Autodesk Inventor part; units mm, degrees
ref_plane "YZ Plane" through (0, 0, 0) normal (1, 0, 0) x (0, 1, 0)
ref_plane "XZ Plane" through (0, 0, 0) normal (0, 1, 0) x (-1, 0, 0)
ref_plane "XY Plane" through (0, 0, 0) normal (0, 0, 1) x (1, 0, 0)
sketch "Sketch1" plane through (0, 0, 0) normal (0, 1, 0) x (-1, 0, 0)
  circle A0 centre (0, 0) radius 27.5
  circle A1 centre (0, 0) radius 12.7
  dimension "d1" = 55
  dimension "d14" = 25.4
extrude "Extrusion1" add sketch "Sketch1" along normal blind 20 contours A0 | A1
extrude "Extrusion2" cut sketch "Sketch1" along normal blind 11.4 contours A1
sketch "Sketch2" plane through (0, 11.4, 0) normal (0, -1, 0) x (1, 0, 0)
  circle A0 centre (0, 0) radius 5.2
  dimension "d17" = 10.4
chamfer "Chamfer2" distance 11.4 distance2 7.5 1 edges at (12.7, 11.4, 0) measured on face at (-12.5355, 7.6, -2.0372)
extrude "Extrusion3" cut sketch "Sketch2" against normal blind 11.4
properties part number "2. ring"
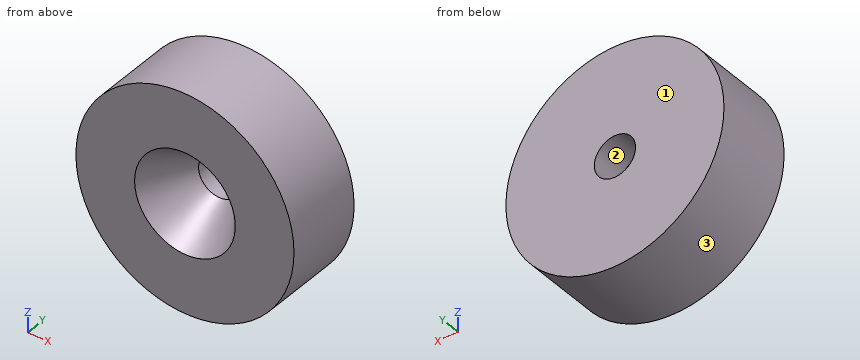
Build history of the part. All positions in model axes, mm. Face numbers are marked on the shaded views. Coordinates: 2 decimals unless noted, no trailing zeros. Write each loop counter-clockwise with the first axis right and the second up, starting at its lowest first coordinate (ties: lowest second). Pieces come first, ordered by that corner, then holes.
(1) Drill centre lines: line 1 (Z direction, x = 0, y = 14); line 2 (Z direction, x = 0, y = 0.05); line 3 (X direction, y = 3.5, z = -6). Where is each one in solid material? Low to high.
(2) Pin check, flat tips, straight feed: pin 1 Ø6 at (x, y) = (-2.5, 4) entering from -Z; pin 2 Ø12 at (x, z) = (0, 0) entering from -Y; pin 3 Ø3 at (x, y) = (13, 10.5) entering from +Z; pin 4 Ø5 at (x, z) = (-2, 1) entering from -Y. Stop position of each tip, or through.
(3) Mould opens along X. For the marked faces 1, 2 and 3 say: pulls with the +X half, pulls with the -X half, needs draft (parallel to the pull), parting line crosses it, or undercut.
(4) Cut at C-C on y = 12.75. List the corners of the cut face in (x, z), and give its area (3 significant figures).
(5) Cut at D-D on x = -23.5. List the corners of the cut face in (y, z).
Working result:
1. line 1: z = -27.5 to -5.2, 5.2 to 27.5
1. line 2: z = -27.5 to -12.67, 12.67 to 27.5
1. line 3: x = -26.84 to -8.49, 8.49 to 26.84
2. pin 1: stops at z = -27.5
2. pin 2: stops at y = 10.18
2. pin 3: stops at z = 24.98
2. pin 4: passes through
3. face 1: needs draft
3. face 2: undercut
3. face 3: parting line crosses it
4. outline: circle Ø55 at (0, 0); hole circle Ø10.4 at (0, 0)
4. area: 2,290 mm2
5. outline: (0, -14.28) - (20, -14.28) - (20, 14.28) - (0, 14.28) - close
